from build123d import *

# Parameters (mm, degrees)
SKETCH012_R   = 100
SKETCH012_R_2 = 10
PAD009_DEPTH  = 100
SKETCH013_R   = 150
SKETCH013_R_2 = 10
PAD011_DEPTH  = 1
SKETCH014_R   = 150
PAD010_DEPTH  = 1


with BuildPart() as part:
    # Sketch012 → Pad009 (new body)
    with BuildSketch(Plane.YZ):
        Circle(SKETCH012_R)
        Circle(SKETCH012_R_2, mode=Mode.SUBTRACT)
    extrude(amount=PAD009_DEPTH)

    # Sketch013 (on Face3 of Pad009) → Pad011 (join)
    with BuildSketch(Plane(origin=(0, 0, 0), x_dir=(0, 1, 0), z_dir=(-1, 0, 0))):
        Circle(SKETCH013_R)
        Circle(SKETCH013_R_2, mode=Mode.SUBTRACT)
    extrude(amount=PAD011_DEPTH)

    # Sketch014 (on Face3 of Pad011) → Pad010 (join)
    with BuildSketch(Plane.YZ.offset(100)):
        Circle(SKETCH014_R)
    extrude(amount=PAD010_DEPTH)


with BuildPart() as part_1:
    # Body004 placement: moved
    add(part.part.moved(Location((112, -225, 160))))


solid = part_1.part
Model file for the job. Use its own axes, mm. A direction names the side the tool comes from. Round coordinates to 2 decimals unless told otherwise and drop trailing zeros. Loops run counter-clockwise (first coordinate to the right, second up) from the corner with the lowest first, then second, coordinate; pieces in that order, holes last. Notation, with made-up numbers: M 77,54 L 92,54 A21 cw 92,73 Z; hole C 66.25,-6 d5. An arc over 180 degrees is marked long. One line per question, with ' | ' between items.
1) Band-saw the part on A-A (y = -225). Give the cut face in (x, z), then the cut area to 3 significant figures.
Solved:
outline: M 111,10 L 112,10 L 112,60 L 212,60 L 212,10 L 213,10 L 213,310 L 212,310 L 212,260 L 112,260 L 112,310 L 111,310 L 111,170 L 212,170 L 212,150 L 111,150 Z | area: 18,600 mm²
2) Band-saw the part on D-D (x = 126.5). Give the cut face in (y, z).
Solved:
outline: C -225,160 d200; hole C -225,160 d20
3) Band-saw the part on C-C (z = 127). Give the cut face in (x, y), then the cut area to 3 significant figures.
Solved:
outline: M 111,-371.32 L 112,-371.32 L 112,-319.4 L 212,-319.4 L 212,-371.32 L 213,-371.32 L 213,-78.68 L 212,-78.68 L 212,-130.6 L 112,-130.6 L 112,-78.68 L 111,-78.68 Z | area: 19,500 mm²
4) Band-saw the part on B-B (z = 276.5). Give the cut face in (x, y).
Solved:
outline: M 111,-319.49 L 112,-319.49 L 112,-130.51 L 111,-130.51 Z; M 212,-319.49 L 213,-319.49 L 213,-130.51 L 212,-130.51 Z
5) Drill centre lines: line 1 along X through (y, z) = (-265, 278); line 2 along Z through (x, y) = (178, -225); line 3 along Y through (x, z) = (192, 154). Where is each one in solid material? Low to high.
Solved:
line 1: x = 111 to 112, 212 to 213 | line 2: z = 60 to 150, 170 to 260 | line 3: y = -324.82 to -233, -217 to -125.18
6) Mould opens along Z. For faces 1 (the cylindrical face through (162.207, -215.763, 163.83)), 2 (the cylindrical face through (212.493, -86.438, 102.549)), 3 (the flat face through (212, -225, 160)), 4 (the flat face through (213, -227, 162)) say: +Z half, -Z half, draft (parallel to the pull), parting line (faces both ways), or undercut.
Solved:
face 1: undercut | face 2: parting line | face 3: undercut | face 4: draft
7) 3-axis set-ups, long thin cutter, end or side, ignore diameter. For faces 5 (the flat face through (112, -194, 258)), 6 (the flat face through (111, -194, 158)): which of +Z, -Z, +X, -X, +Y, -Y reach the whole face in a straight line?
Solved:
face 5: none | face 6: +Z, -Z, -X, +Y, -Y
8) Flat gauge pins, fed straight in: pin 1 (4 mm diameter, centred on x = 179, z = 67.5, fed in from -Y); pin 2 (2 mm diameter, centred on x = 186, y = -282, fed in from -Z); pin 3 (1 mm diameter, centred on x = 169.5, z = 201.5, fed in from +Y). Where does each tip first touch, or does it go through?
Solved:
pin 1: stops at y = -267.54 | pin 2: stops at z = 77.15 | pin 3: stops at y = -133.79
